Build history of the part. All positions in model axes, mm. A direction names the side the tool comes from. Give positions to 0.01 mm unless a question says otherwise; leave off trailing zeros. Order: outer loops, then holes, each group sorted by start corner. A loop starts at its lowest first (then second) coordinate and runs counter-clockwise, first axis right, second up. Notation, with made-up numbers: M -20.75,63 L 33.25,63 A24 ccw 33.25,100 Z; hole C 67,38.5 d4. An arc over 180 degrees is marked long. One line per item, written item: value.
from build123d import *

# Parameters (mm, degrees)
SKETCH1_W           = 17.5006
SKETCH1_H           = 5.7658
BOSS_EXTRUDE1_DEPTH = 6.985
SKETCH2_W           = 0.6604
SKETCH2_H           = 0.6604
BOSS_EXTRUDE2_DEPTH = 3.175
SKETCH4_W           = 16.2306
SKETCH4_H           = 4.4958
CUT_EXTRUDE1_DEPTH  = 6.35
SKETCH2_2_W         = 0.6604
SKETCH2_2_H         = 0.6604
BOSS_EXTRUDE3_DEPTH = 6.35
SKETCH5_W           = 0.635
SKETCH5_H           = 1.016
SKETCH5_W_2         = 1.524
SKETCH5_H_2         = 0.635
CUT_EXTRUDE2_DEPTH  = 3.556


with BuildPart() as part:
    # Sketch1 → Boss-Extrude1 (new body)
    with BuildSketch(Plane.XY):
        with Locations((8.7503, 2.8829)):
            Rectangle(SKETCH1_W, SKETCH1_H)
    extrude(amount=BOSS_EXTRUDE1_DEPTH)

    # Sketch2 → Boss-Extrude2 (add)
    with BuildSketch(Plane(origin=(0, 0, 0), x_dir=(-1, 0, 0), z_dir=(0, 0, -1))):
        with Locations((-12.5003, 3.4036)):
            Rectangle(SKETCH2_W, SKETCH2_H)
        with Locations((-10.0003, 3.4036)):
            Rectangle(SKETCH2_W, SKETCH2_H)
        with Locations((-7.5003, 3.4036)):
            Rectangle(SKETCH2_W, SKETCH2_H)
        with Locations((-5.0003, 3.4036)):
            Rectangle(SKETCH2_W, SKETCH2_H)
        with Locations((-15.0003, 3.4036)):
            Rectangle(SKETCH2_W, SKETCH2_H)
        with Locations((-2.5003, 3.4036)):
            Rectangle(SKETCH2_W, SKETCH2_H)
    extrude(amount=BOSS_EXTRUDE2_DEPTH)

    # Sketch4 → Cut-Extrude1 (cut)
    with BuildSketch(Plane.XY.offset(6.985)):
        with Locations((8.7503, 2.8829)):
            Rectangle(SKETCH4_W, SKETCH4_H)
    extrude(amount=-CUT_EXTRUDE1_DEPTH, mode=Mode.SUBTRACT)

    # Sketch2<2> → Boss-Extrude3 (add)
    with BuildSketch(Plane(origin=(0, 0, 0), x_dir=(-1, 0, 0), z_dir=(0, 0, -1))):
        with Locations((-12.5003, 3.4036)):
            Rectangle(SKETCH2_2_W, SKETCH2_2_H)
        with Locations((-10.0003, 3.4036)):
            Rectangle(SKETCH2_2_W, SKETCH2_2_H)
        with Locations((-7.5003, 3.4036)):
            Rectangle(SKETCH2_2_W, SKETCH2_2_H)
        with Locations((-5.0003, 3.4036)):
            Rectangle(SKETCH2_2_W, SKETCH2_2_H)
        with Locations((-15.0003, 3.4036)):
            Rectangle(SKETCH2_2_W, SKETCH2_2_H)
        with Locations((-2.5003, 3.4036)):
            Rectangle(SKETCH2_2_W, SKETCH2_2_H)
    extrude(amount=-BOSS_EXTRUDE3_DEPTH)

    # Sketch5 → Cut-Extrude2 (cut)
    with BuildSketch(Plane.XY.offset(6.985)):
        with Locations((0.3175, 4.3688)):
            Rectangle(SKETCH5_W, SKETCH5_H)
        with Locations((17.1831, 4.3688)):
            Rectangle(SKETCH5_W, SKETCH5_H)
        with Locations((14.8463, 5.4483)):
            Rectangle(SKETCH5_W_2, SKETCH5_H_2)
        with Locations((2.6543, 5.4483)):
            Rectangle(SKETCH5_W_2, SKETCH5_H_2)
    extrude(amount=-CUT_EXTRUDE2_DEPTH, mode=Mode.SUBTRACT)


solid = part.part
1) Mould opens along Y. For faces 1 (the face through (16.866, 3, 4)), 2 (the face through (9, 5.766, 3)), 3 (the face through (0, 3, 3)) say: released by +Y, released by -Y, zero draft, split by the parting line, or undercut.
Check values:
face 1: undercut
face 2: released by +Y
face 3: zero draft
2) Tool access for faces 4 (the face through (8.7, 0.4, 6.985)), 5 (the face through (9, 5.131, 4)): list every direction of +Z, -Z, +X, -X, +Y, -Y with a clear straight run to the whole face (end or side of a thin tool).
Check values:
face 4: +Z, +X, -X, +Y, -Y
face 5: +Z
3) Drill centre lines: probe 1 along X at (y, z) = (3.55, -1.5); probe 2 along X at (y, z) = (5, 1) (3 decimals); probe 3 along Y at (x, z) = (7, 4.75) (3 decimals). Where is each one in solid material? Low to high. Write a range as from..to.
Check values:
probe 1: 2.17..2.83, 4.67..5.33, 7.17..7.83, 9.67..10.33, 12.17..12.83, 14.67..15.33
probe 2: 0..0.635, 16.866..17.501
probe 3: 0..0.635, 5.131..5.766
4) Saw through at A-A, the plane z = -0.5. Write the cut outline in (x, y).
Check values:
outline: M 2.17,3.07 L 2.83,3.07 L 2.83,3.73 L 2.17,3.73 Z; M 4.67,3.07 L 5.33,3.07 L 5.33,3.73 L 4.67,3.73 Z; M 7.17,3.07 L 7.83,3.07 L 7.83,3.73 L 7.17,3.73 Z; M 9.67,3.07 L 10.33,3.07 L 10.33,3.73 L 9.67,3.73 Z; M 12.17,3.07 L 12.83,3.07 L 12.83,3.73 L 12.17,3.73 Z; M 14.67,3.07 L 15.33,3.07 L 15.33,3.73 L 14.67,3.73 Z
5) Saw through at C-C, the plane y = 2.1. Write the cut outline in (x, z) (3 decimals).
Check values:
outline: M 0,0 L 17.501,0 L 17.501,6.985 L 16.866,6.985 L 16.866,0.635 L 0.635,0.635 L 0.635,6.985 L 0,6.985 Z
6) Saw through at B-B, the plane x = 8.5. Write the cut outline in (y, z) (3 decimals), then the cut area to 3 significant figures.
Check values:
outline: M 0,0 L 5.766,0 L 5.766,6.985 L 5.131,6.985 L 5.131,0.635 L 0.635,0.635 L 0.635,6.985 L 0,6.985 Z
area: 11.7 mm^2
7) Saw through at D-D, the plane z = 4. Give the number of separate pieces and of enclosed holes in the cut face, then the cut area to 3 significant figures.
Check values:
separate pieces: 10
enclosed holes: 0
area: 27.3 mm^2
8) Pin check, flat tips, straight feed: pin 1 (0.7 mm diameter, centred on x = 3, y = 5.5, fed in from +Z); pin 2 (0.7 mm diameter, centred on x = 10, y = 3.5, fed in from +Z). Stop position of each tip, or through.
Check values:
pin 1: z = 3.43
pin 2: z = 6.35
